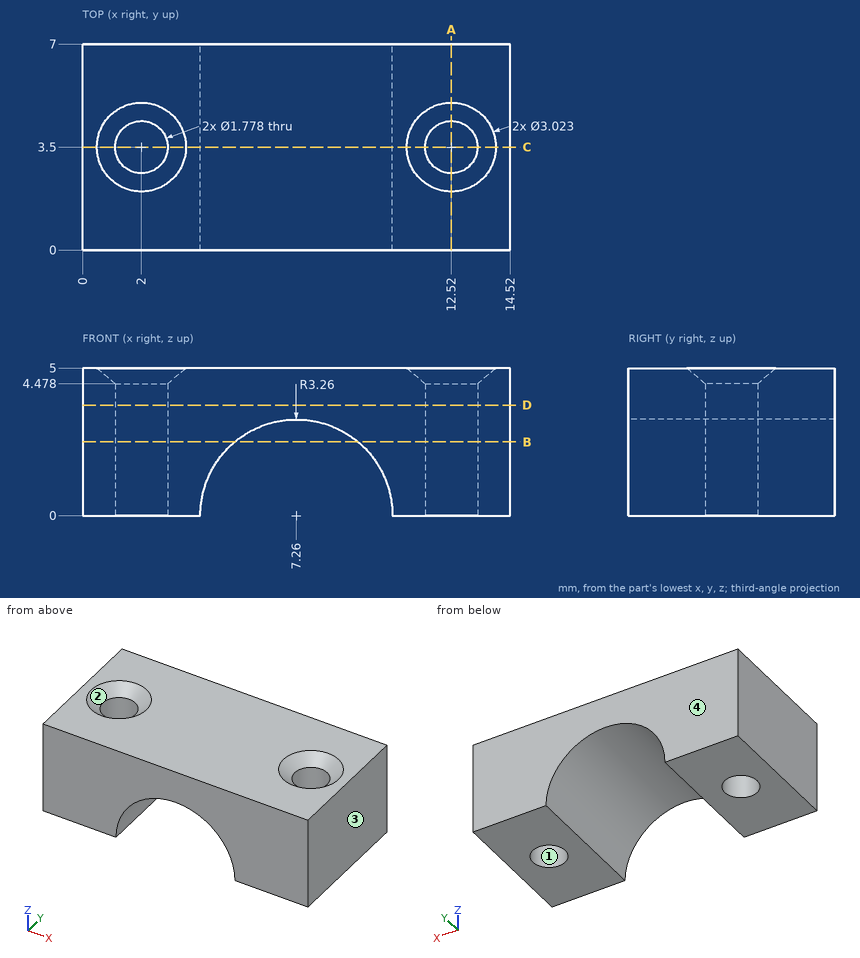
Design review of the part shown in the three views and the two pictorial views. Dimensions are in mm from the part's minimum x, y and z. Give positions to 0.01 mm unless a question says otherwise; leave off trailing zeros. Loops run counter-clockwise (first coordinate to the right, second up) from the corner with the lowest first, then second, coordinate; pieces in that order, holes last. Notation, with made-up numbers: M -29,61 L 12,61 A21 ccw 12,69 Z; hole C 59,78.5 d9. An arc over 180 degrees is marked long. Write item = value, one per line.
Q1. We need section C-C (y = 3.5). Give the boundary of the cut face in (x, z).
Output values:
outline = M 0,0 L 1.11,0 L 1.11,4.48 L 0.49,5 L 0,5 Z; M 2.89,0 L 4,0 A3.26 cw 10.52,0 L 11.63,0 L 11.63,4.48 L 11.01,5 L 3.51,5 L 2.89,4.48 Z; M 13.41,0 L 14.52,0 L 14.52,5 L 14.03,5 L 13.41,4.48 Z
Q2. Draft analysis for pull direction Y (two halves, no side actions). For the marked faces 1, 2, 3 and 4, state which applies: +Y half, -Y half, draft (parallel to the pull), parting line (faces both ways), or undercut.
Output values:
face_1 = undercut
face_2 = undercut
face_3 = draft
face_4 = +Y half
Q3. To check wall thickness, follow line 1 (Y direction, x = 2, z = 1.9); line 2 (X direction, y = 3.5, z = 3.35); line 3 (X direction, y = 3.5, z = 2.65). State the ranges of each line that lie inside material, in increasing order. Write a range as [from, to].
Output values:
line_1 = [0, 2.61], [4.39, 7]
line_2 = [0, 1.11], [2.89, 11.63], [13.41, 14.52]
line_3 = [0, 1.11], [2.89, 5.36], [9.16, 11.63], [13.41, 14.52]
Q4. Insertion check: pin 1 (1.1 mm diameter, centred on x = 12.52, y = 3.5, fed in from -Z). The pin has a flat end and moves straight along its axis. Give the tip position at first contact, or say it passes through.
Output values:
pin_1 = through
Q5. We need section D-D (z = 3.75). Give the boundary of the cut face in (x, y).
Output values:
outline = M 0,0 L 14.52,0 L 14.52,7 L 0,7 Z; hole C 2,3.5 d1.78; hole C 12.52,3.5 d1.78
Q6. We need section B-B (z = 2.5). Give the boundary of the cut face in (x, y).
Output values:
outline = M 0,0 L 5.17,0 L 5.17,7 L 0,7 Z; M 9.35,0 L 14.52,0 L 14.52,7 L 9.35,7 Z; hole C 2,3.5 d1.78; hole C 12.52,3.5 d1.78
Q7. We need section A-A (x = 12.52). Give the boundary of the cut face in (y, z).
Output values:
outline = M 0,0 L 2.61,0 L 2.61,4.48 L 1.99,5 L 0,5 Z; M 4.39,0 L 7,0 L 7,5 L 5.01,5 L 4.39,4.48 Z
